Autodesk Inventor part; units mm, degrees
ref_plane "YZ Plane" through (0, 0, 0) normal (1, 0, 0) x (0, 1, 0)
ref_plane "XZ Plane" through (0, 0, 0) normal (0, 1, 0) x (-1, 0, 0)
ref_plane "XY Plane" through (0, 0, 0) normal (0, 0, 1) x (1, 0, 0)
sketch "Sketch1" plane through (0, 0, 0) normal (0, 0, 1) x (1, 0, 0)
  line L0 (-14, -7) -> (14, -7)
  line L1 (14, -7) -> (14, 7)
  line L2 (14, 7) -> (-14, 7)
  line L3 (-14, 7) -> (-14, -7)
  line L4 (-14, -7) -> (14, 7) construction
  line L5 (14, -7) -> (-14, 7) construction
  point P0 (0, 0)
  dimension "d0" = 14
  dimension "d1" = 28
extrude "Extrusion1" add sketch "Sketch1" along normal blind 30
sketch "Sketch2" plane through (-14, -7, 0) normal (0, -1, 0) x (1, 0, 0)
  line L0 (-6, 15) -> (34, 15) construction
  line L1 (28, 30) -> (0, 30)
  line L2 (-6, 5) -> (34, 5)
  line L3 (34, 25) -> (-6, 25)
  arc A0 (-6, 25) -> (-6, 5) centre (-6, 15) ccw
  arc A1 (34, 5) -> (34, 25) centre (34, 15) ccw
  line L4 (14, 15) -> (14, 0) construction
  circle A2 centre (-6, 15) radius 3
  circle A3 centre (34, 15) radius 3
  line L5 (28, 0) -> (0, 0)
  dimension "d4" = 40
  dimension "d5" = 10
  dimension "d8" = 6
  dimension "d17" = 15
extrude "Extrusion2" add sketch "Sketch2" against normal blind 4
sketch "Sketch3" plane through (-14, 7, 0) normal (0, 1, 0) x (1, 0, 0)
  line L0 (28, 0) -> (0, 0) construction
  line L1 (0, 0) -> (0, -30) construction
  line L2 (28, -30) -> (0, -30) construction
  line L3 (28, 0) -> (28, -30) construction
  line L4 (3, -27) -> (3, -3) construction
  line L5 (3, -3) -> (25, -3) construction
  line L6 (25, -3) -> (25, -27) construction
  line L7 (25, -27) -> (3, -27) construction
  circle A0 centre (25, -27) radius 1.75
  circle A1 centre (3, -27) radius 1.75
  circle A2 centre (3, -3) radius 1.75
  circle A3 centre (25, -3) radius 1.75
  point P0 (14, 0)
  dimension "d9" = 22
  dimension "d10" = 24
  dimension "d11" = 3.5
extrude "Extrusion3" cut sketch "Sketch3" against normal through all
sketch "Sketch4" plane through (-14, -7, 0) normal (0, -1, 0) x (1, 0, 0)
  circle A0 centre (25, 27) radius 1.75
  circle A1 centre (25, 27) radius 3
  circle A2 centre (25, 3) radius 1.75
  circle A3 centre (25, 3) radius 3
  circle A4 centre (3, 3) radius 1.75
  circle A5 centre (3, 3) radius 3
  circle A6 centre (3, 27) radius 1.75
  circle A7 centre (3, 27) radius 3
  circle A8 centre (25, 27) radius 1.75
  circle A9 centre (25, 3) radius 1.75
  circle A10 centre (3, 3) radius 1.75
  circle A11 centre (3, 27) radius 1.75
  circle A12 centre (-6, 15) radius 3
  circle A13 centre (34, 15) radius 3
  line L0 (0, 0) -> (0, 5)
  line L1 (0, 0) -> (28, 0)
  line L2 (28, 0) -> (28, 5)
  line L3 (28, 5) -> (34, 5)
  arc A14 (34, 5) -> (34, 25) centre (34, 15) ccw
  line L4 (0, 30) -> (28, 30)
  arc A15 (-6, 25) -> (-6, 5) centre (-6, 15) ccw
  line L5 (-6, 5) -> (0, 5)
  line L6 (28, 25) -> (28, 30)
  line L7 (0, 25) -> (0, 30)
  line L8 (0, 25) -> (-6, 25)
  line L9 (34, 25) -> (28, 25)
  point P0 (14, 0)
  point P1 (0, 3)
  point P2 (3, 0)
  point P3 (28, 3)
  point P4 (25, 0)
  point P5 (0, 27)
  point P6 (3, 30)
  point P7 (28, 27)
  point P8 (25, 30)
  dimension "d14" = 6
extrude "Extrusion4" cut sketch "Sketch4" against normal blind 5 contours A1 | A1 L4 L6 | A7 | A7 L7 L4 | A3 | L2 L1 A3 | L1 L0 A5 | A5
properties part number "StantonBracket"
Geometry: final body of the model. Coordinates: model frame, mm. A direction names the side the tool comes from. Give positions to 0.01 mm unless a question says otherwise; leave off trailing zeros. Write each loop counter-clockwise with the first axis right and the second up, starting at its lowest first coordinate (ties: lowest second). Pieces come first, ordered by that corner, then holes.
1. Section query B-B, the plane z = 17.25. Return loops of the section in (x, y).
2. Section query A-A, the plane y = 6.25. Return loops of the section in (x, z), then the cut area to 3 significant figures.
3. Pin query (flat end, axial travel): P1, Ø1.2, axis at x = 15.5, y = -5, coming from the -Z side; P2, Ø3, axis at x = -12, z = 28, coming from the -Y side; P3, Ø8, axis at x = 21.5, z = 17.5, coming from the +Y side. Return the tip coordinate at first contact, or that it passes through.
4. Reachability of faces 5 (the flat face through (-17, -5, 25)), 6 (the flat face through (17, -5, 25)), 7 (the flat face through (24, -3, 15)) from +Z, -Z, +X, -X, +Y, -Y: full face, straight path, thin tool, end or side. Return the list, or none.
5. Section query D-D, the plane z = 20.75. Return loops of the section in (x, y).
6. Draft query along Z for faces 1 (the flat face through (14, 1, 15)), 2 (the flat face through (0, 0, 30)), 3 (the cylindrical face through (-9.383, 2.563, 3.67)), 4 (the flat face through (-12.4, -2, 1.7)). Return one class per face: released by +Z, released by -Z, zero draft, split by the parting line, or undercut.
7. Line query: probe 1 along Z at (x, y) = (11, 2); probe 2 along Z at (x, y) = (20, -3.85); probe 3 along X at (y, z) = (-5.75, 12.75). Output: solid intervals per line, ascending.
8. Section query C-C, the plane x = -26. Return loops of the section in (y, z), then the cut area to 3 significant figures.
Computed:
1. outline: (-29.74, -7) - (-21.98, -7) - (-21.98, -3) - (-29.74, -3) - close; (-18.02, -7) - (18.02, -7) - (18.02, -3) - (14, -3) - (14, 7) - (-14, 7) - (-14, -3) - (-18.02, -3) - close; (21.98, -7) - (29.74, -7) - (29.74, -3) - (21.98, -3) - close
2. outline: (-14, 0) - (14, 0) - (14, 30) - (-14, 30) - close; hole circle Ø3.5 at (-11, 3); hole circle Ø3.5 at (-11, 27); hole circle Ø3.5 at (11, 3); hole circle Ø3.5 at (11, 27)
2. area: 802 mm2
3. P1: stops at z = 5
3. P2: stops at y = -2
3. P3: stops at y = -3
4. face 5: +Z, -X, +Y, -Y
4. face 6: +Z, +X, +Y, -Y
4. face 7: +Z, -Z, +X, +Y
5. outline: (-28.18, -7) - (28.18, -7) - (28.18, -3) - (14, -3) - (14, 7) - (-14, 7) - (-14, -3) - (-28.18, -3) - close
6. face 1: zero draft
6. face 2: released by +Z
6. face 3: undercut
6. face 4: undercut
7. probe 1: z = 0 to 1.25, 4.75 to 25.25, 28.75 to 30
7. probe 2: z = 5 to 12, 18 to 25
7. probe 3: x = -29.74 to -21.98, -18.02 to 18.02, 21.98 to 29.74
8. outline: (-7, 7) - (-3, 7) - (-3, 23) - (-7, 23) - close
8. area: 64.0 mm2
